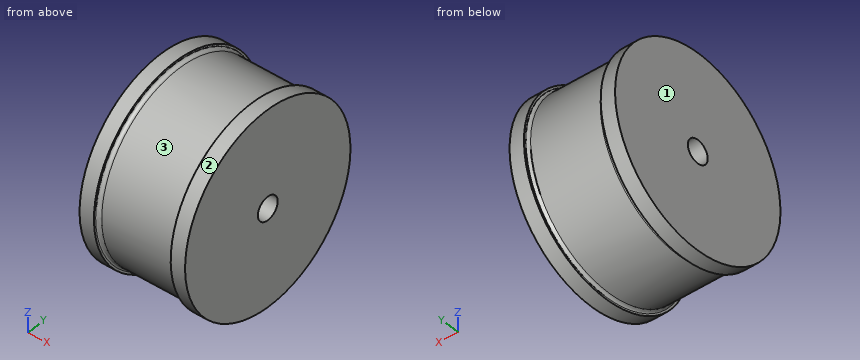
```python
from build123d import *

# Parameters (mm, degrees)
SKETCH3_R          = 6
CUT_EXTRUDE1_DEPTH = 104.136405777


with BuildPart() as part:
    # Sketch1 → Revolve1 (revolve)
    with BuildSketch(Plane.XY, mode=Mode.PRIVATE) as revolve1_sk:
        with BuildLine():
            Line((23.876500295, 28.500921708), (23.876500295, -21.499078292))
            Line((23.876500295, -21.499078292), (19.38343903, -21.499078292))
            Line((19.38343903, -21.499078292), (-23.623499705, -21.499078292))
            Line((-23.623499705, -21.499078292), (-31.123499705, -21.499078292))
            Line((-31.123499705, -21.499078292), (-31.123499705, 20.226597036))
            Line((-31.123499705, 20.226597036), (-31.123499705, 28.500921708))
            Line((-31.123499705, 28.500921708), (-23.623499705, 28.500921708))
            Line((-23.623499705, 28.500921708), (-23.623499705, 27.45743453))
            ThreePointArc((-23.623499705, 27.45743453), (-22.782204784, 26.431489238), (-21.461866567, 26.300921708))
            Line((-21.461866567, 26.300921708), (-3.623499705, 26.300921708))
            Line((-3.623499705, 26.300921708), (14.814368071, 26.300921708))
            ThreePointArc((14.814368071, 26.300921708), (15.776775387, 26.633474133), (16.376500295, 27.456364765))
            Line((16.376500295, 27.456364765), (16.376500295, 28.500921708))
            Line((16.376500295, 28.500921708), (23.876500295, 28.500921708))
        make_face()
    revolve(revolve1_sk.sketch.rotate(Axis((23.876500295, -21.499078292, 0), (-1, 0, 0)), 90), axis=Axis((23.876500295, -21.499078292, 0), (-1, 0, 0)))

    # Sketch3 → Cut-Extrude1 (cut, through all)
    with BuildSketch(Plane(origin=(23.876500295, 0, 0), x_dir=(0, 0, -1), z_dir=(1, 0, 0))):
        with Locations((0, -21.499078292)):
            Circle(SKETCH3_R)
    extrude(amount=-CUT_EXTRUDE1_DEPTH, mode=Mode.SUBTRACT)


solid = part.part
```
Can you work these out from the model? Positions are in its coordinate system, mm. Face numbers are marked on the shaded views. Coordinates: 2 decimals unless noted, no trailing zeros. Write each loop counter-clockwise with the first axis right and the second up, starting at its lowest first coordinate (ties: lowest second). Pieces come first, ordered by that corner, then holes. Notation, with made-up numbers: (-31.75, 46) - (-27.75, 46) arc R22 cw to (-27.75, 77) - close; hole circle Ø11 at (26.25, 69.25). An arc over 180 degrees is marked (long way). Return JSON: item names as keys, results as strings.
Q1. I'm going to push flat-ended pins straight in: pin 1 Ø1 at (x, z) = (14.5, -30.5) entering from +Y; pin 2 Ø10 at (x, z) = (-10.5, -30.5) entering from -Y; pin 3 Ø1.5 at (x, z) = (10.5, -34.5) entering from +Y. Where does each tip first touch, or does it pass through?
Computed values:
{"pin 1": "stops at y = 15.71", "pin 2": "stops at y = -61.93", "pin 3": "stops at y = 12.35"}
Q2. If we section it at A-A (z = 0): Please give me the cut outline in (x, y), then the cut area to 3 significant figures.
Computed values:
{"outline": "(-31.12, -71.5) - (-23.62, -71.5) - (-23.62, -70.46) arc R1.73 cw to (-21.46, -69.3) - (14.81, -69.3) arc R1.7 cw to (16.38, -70.45) - (16.38, -71.5) - (23.88, -71.5) - (23.88, -27.5) - (-31.12, -27.5) - close; (-31.12, -15.5) - (23.88, -15.5) - (23.88, 28.5) - (16.38, 28.5) - (16.38, 27.46) arc R1.7 cw to (14.81, 26.3) - (-21.46, 26.3) arc R1.73 cw to (-23.62, 27.46) - (-23.62, 28.5) - (-31.12, 28.5) - close", "area": "4,670 mm2"}
Q3. If we section it at B-B (x = 11.5): Please give me the cut outline in (y, z).
Computed values:
{"outline": "circle Ø95.6 at (-21.5, 0); hole circle Ø12 at (-21.5, 0)"}
Q4. Please list where these lines run through material, in increasing order: L1, parallel to Y at x = -5.5, z = 0; L2, parallel to Z at x = -6.5, y = -21; L3, parallel to Z at x = -23, y = -20.5. Write a range as from..to.
Computed values:
{"L1": "y = -69.3..-27.5, -15.5..26.3", "L2": "z = -47.8..-5.98, 5.98..47.8", "L3": "z = -48.06..-5.92, 5.92..48.06"}
Q5. Thinking about a two-plate mould opening in X: for the marked faces 1, 2 and 3, which applies, +X half, -X half, draft (parallel to the pull), parting line (faces both ways), or undercut?
Computed values:
{"face 1": "-X half", "face 2": "draft", "face 3": "undercut"}
